CAD build for the part. Positions are in the model's coordinates, mm. Face numbers are marked on the shaded views. A direction names the side the tool comes from. Give positions to 0.01 mm unless a question says otherwise; leave off trailing zeros. Order: outer loops, then holes, each group sorted by start corner. A loop starts at its lowest first (then second) coordinate and runs counter-clockwise, first axis right, second up.
Item 1: Wall check: L1, parallel to X at y = -12.5, z = 3.7; L2, parallel to Y at x = 32.5, z = 2.2; L3, parallel to X at y = 2.5, z = 4.2. Give the ranges that are in metal, low to high.
Item 2: Band-saw the part on B-B on x = 32.5. Give the cut face in (y, z).
Item 3: Flat gauge pins, fed straight in: P1, Ø3, axis at y = 10.5, z = 1.5, coming from the +X side; P2, Ø8, axis at x = 6.5, y = 13.5, coming from the +Z side. Where does each tip first touch, or does it go through?
Item 4: Band-saw the part on C-C on x = -27.5. Give the cut face in (y, z).
Item 5: Band-saw the part on D-D on y = -12.5. Give the cut face in (x, z), plus the area to 3 significant figures.
Item 6: Which spindle directions (+Z, -Z, +X, -X, +Y, -Y) get a long thin tool onto all of the face, cutting with end or side? Do the marked faces 1 and 2. Say none if no direction does.
Item 7: Band-saw the part on A-A on y = 2.5. Give the cut face in (x, z).
Solid Edge part; units mm, degrees
sketch "Sketch1" plane through (0, 0, 0) normal (0, 0, 1) x (1, 0, 0)
  line L0 (37.5, -17.5) -> (-37.5, -17.5)
  line L1 (-37.5, -17.5) -> (-37.5, 17.5)
  line L2 (-37.5, 17.5) -> (37.5, 17.5)
  line L3 (37.5, 17.5) -> (37.5, -17.5)
  dimension "D1" = 37.5
  dimension "D2" = 37.5
extrude "Protrusion1" add sketch "Sketch1" along normal blind 5.5
hole "Hole_1" at (32.5, -12.5, 5.5) direction (0, 0, -1) diameter 3.2 end up to next
sketch "Sketch2" plane through (0, 0, 5.5) normal (0, 0, 1) x (1, 0, 0)
  line L0 (-22.5, 17.5) -> (-22.5, 7.5)
  line L1 (-22.5, 7.5) -> (37.5, 7.5)
  dimension "D1" = 22.5
extrude "Cutout1" cut sketch "Sketch2" against normal through all material side at (-22.45, 12.5, 5.5)
hole "Hole_2" at (-33.2785, 11.4414, 5.5) direction (0, 0, -1) diameter 3.2 end up to next
hole "Hole1" at (32.5, 2.5, 5.5) direction (0, 0, -1) diameter 3.2 end up to next
hole "Hole2" at (-27.5, -12.5, 5.5) direction (0, 0, -1) diameter 3.2 end up to next
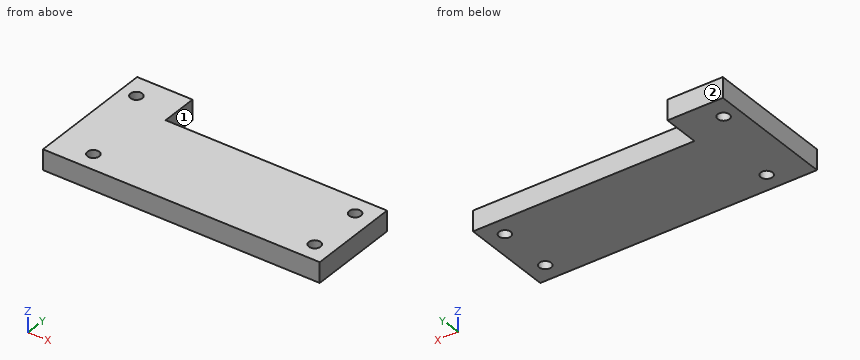
The answers:
1. L1: x = -37.5 to -29.1, -25.9 to 30.9, 34.1 to 37.5
1. L2: y = -17.5 to -14.1, -10.9 to 0.9, 4.1 to 7.5
1. L3: x = -37.5 to 30.9, 34.1 to 37.5
2. outline: (-17.5, 0) - (-14.1, 0) - (-14.1, 5.5) - (-17.5, 5.5) - close; (-10.9, 0) - (0.9, 0) - (0.9, 5.5) - (-10.9, 5.5) - close; (4.1, 0) - (7.5, 0) - (7.5, 5.5) - (4.1, 5.5) - close
3. P1: stops at x = -22.5
3. P2: passes through
4. outline: (-17.5, 0) - (-14.1, 0) - (-14.1, 5.5) - (-17.5, 5.5) - close; (-10.9, 0) - (17.5, 0) - (17.5, 5.5) - (-10.9, 5.5) - close
5. outline: (-37.5, 0) - (-29.1, 0) - (-29.1, 5.5) - (-37.5, 5.5) - close; (-25.9, 0) - (30.9, 0) - (30.9, 5.5) - (-25.9, 5.5) - close; (34.1, 0) - (37.5, 0) - (37.5, 5.5) - (34.1, 5.5) - close
5. area: 377 mm2
6. face 1: +Z, -Z, +X, +Y
6. face 2: +Z, -Z, +X, -X, +Y
7. outline: (-37.5, 0) - (30.9, 0) - (30.9, 5.5) - (-37.5, 5.5) - close; (34.1, 0) - (37.5, 0) - (37.5, 5.5) - (34.1, 5.5) - close
